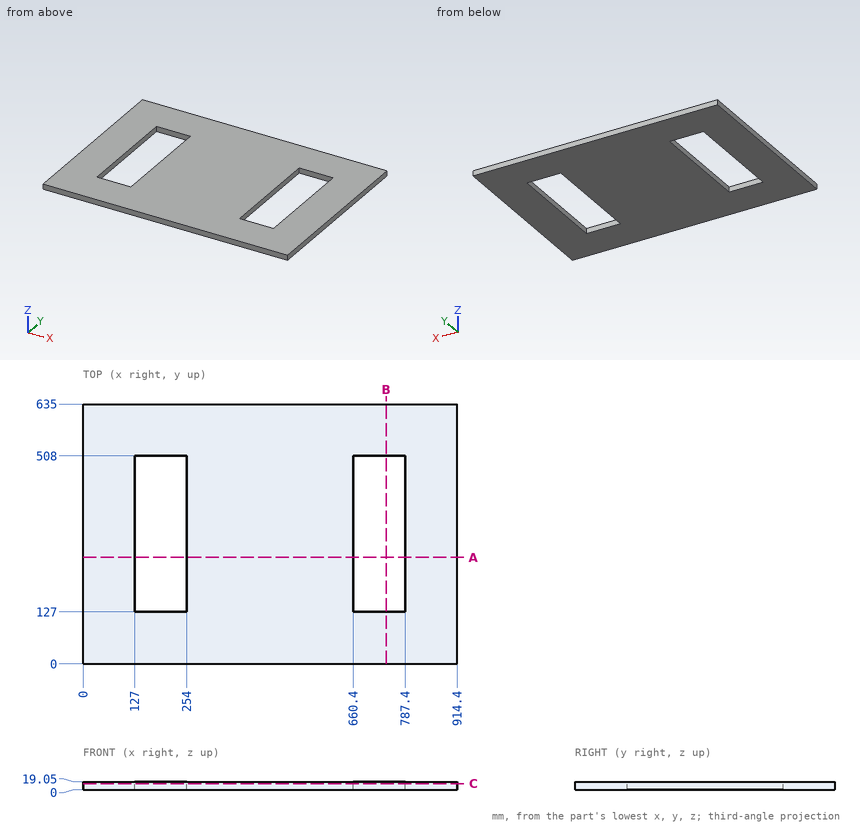
Geometry: see drawing. Coordinates: mm, zero at the bounding-box minimum. Round coordinates to 2 decimals unless told otherwise and drop trailing zeros. Write each loop counter-clockwise with the first axis right and the second up, starting at its lowest first coordinate (ties: lowest second). Pieces come first, ordered by that corner, then holes.
Item 1: Material intervals for L1, parallel to X at y = 456, z = 14.75; L2, parallel to Y at x = 722.5, z = 9.5, sorted ascending.
Item 2: Pin query (flat end, axial travel): P1, Ø3, axis at y = 167, z = 17, coming from the -X side. Return the tip coordinate at first contact, or that it passes through.
Item 3: Section query B-B (x = 740.5). Return loops of the section in (y, z).
Item 4: Section query A-A (y = 260). Return loops of the section in (x, z).
Item 5: Section query C-C (z = 14.5). Return loops of the section in (x, y).
Completed:
1. L1: x = 0 to 127, 254 to 660.4, 787.4 to 914.4
1. L2: y = 0 to 127, 508 to 635
2. P1: stops at x = 0
3. outline: (0, 0) - (127, 0) - (127, 19.05) - (0, 19.05) - close; (508, 0) - (635, 0) - (635, 19.05) - (508, 19.05) - close
4. outline: (0, 0) - (127, 0) - (127, 19.05) - (0, 19.05) - close; (254, 0) - (660.4, 0) - (660.4, 19.05) - (254, 19.05) - close; (787.4, 0) - (914.4, 0) - (914.4, 19.05) - (787.4, 19.05) - close
5. outline: (0, 0) - (914.4, 0) - (914.4, 635) - (0, 635) - close; hole (127, 127) - (254, 127) - (254, 508) - (127, 508) - close; hole (660.4, 127) - (787.4, 127) - (787.4, 508) - (660.4, 508) - close
